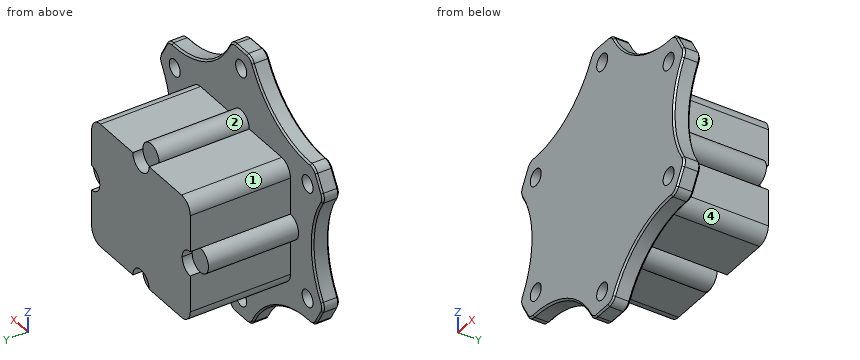
```python
from build123d import *

# Parameters (mm, degrees)
BOSS_EXTRUDE1_DEPTH    = 5
F_10_CLEARANCE_HOLE1_D = 5
FILLET1_R              = 3
CHAMFER1_SIZE          = 0.5
BOSS_EXTRUDE4_DEPTH    = 30
SKETCH5_R              = 3.7
BOSS_EXTRUDE5_DEPTH    = 27


with BuildPart() as part:
    # Sketch1 → Boss-Extrude1 (new body)
    with BuildSketch(Plane.XZ.offset(-227)):
        with BuildLine():
            Line((610.472328875, 48.998023491), (619.472328875, 48.998023491))
            ThreePointArc((619.472328875, 48.998023491), (631.222328875, 61.852197868), (648.22937043, 65.600909174))
            Line((648.22937043, 65.600909174), (652.72937043, 73.395137808))
            ThreePointArc((652.72937043, 73.395137808), (647.472328875, 89.998023491), (652.72937043, 106.600909174))
            Line((652.72937043, 106.600909174), (648.22937043, 114.395137808))
            ThreePointArc((648.22937043, 114.395137808), (631.222328875, 118.143849114), (619.472328875, 130.998023491))
            Line((619.472328875, 130.998023491), (610.472328875, 130.998023491))
            ThreePointArc((610.472328875, 130.998023491), (598.722328875, 118.143849114), (581.71528732, 114.395137808))
            Line((581.71528732, 114.395137808), (577.21528732, 106.600909174))
            ThreePointArc((577.21528732, 106.600909174), (582.472328875, 89.998023491), (577.21528732, 73.395137808))
            Line((577.21528732, 73.395137808), (581.71528732, 65.600909174))
            ThreePointArc((581.71528732, 65.600909174), (598.722328875, 61.852197868), (610.472328875, 48.998023491))
        make_face()
    extrude(amount=-BOSS_EXTRUDE1_DEPTH)

    # #10 Clearance Hole1 (through all)
    with Locations(Plane(origin=(0, 232, 0), x_dir=(1, 0, 0), z_dir=(0, 1, 0))):
        with Locations((614.972328875, -124.998023491), (584.661439743, -72.498023491), (584.661439743, -107.498023491), (614.972328875, -54.998023491), (645.283218008, -107.498023491), (645.283218008, -72.498023491)):
            Hole(F_10_CLEARANCE_HOLE1_D / 2)

    # Fillet1
    fillet1_edges = [part.edges().sort_by_distance(p)[0] for p in [
        (581.71528732, 229.5, 65.600909174),
        (577.21528732, 229.5, 73.395137808),
        (577.21528732, 229.5, 106.600909174),
        (581.71528732, 229.5, 114.395137808),
        (610.472328875, 229.5, 130.998023491),
        (619.472328875, 229.5, 130.998023491),
        (648.22937043, 229.5, 114.395137808),
        (652.72937043, 229.5, 106.600909174),
        (652.72937043, 229.5, 73.395137808),
        (648.22937043, 229.5, 65.600909174),
        (619.472328875, 229.5, 48.998023491),
        (610.472328875, 229.5, 48.998023491),
    ]]
    fillet(fillet1_edges, radius=FILLET1_R)

    # Chamfer1
    chamfer1_edges = [part.edges().sort_by_distance(p)[0] for p in [
        (647.472328875, 227, 89.998023491),
        (647.472328875, 232, 89.998023491),
        (598.722328875, 227, 61.852197868),
        (614.972328875, 227, 48.998023491),
        (631.222328875, 227, 61.852197868),
        (650.47937043, 227, 69.498023491),
        (650.47937043, 227, 110.498023491),
        (631.222328875, 227, 118.143849114),
        (614.972328875, 227, 130.998023491),
        (598.722328875, 227, 118.143849114),
        (579.46528732, 227, 110.498023491),
        (582.472328875, 227, 89.998023491),
        (579.46528732, 227, 69.498023491),
        (581.92524679, 227, 113.911492617),
        (610.786198162, 227, 130.57437066),
        (610.786198162, 227, 49.421676322),
        (577.739116077, 227, 73.335145448),
        (619.158459588, 227, 49.421676322),
        (648.01941096, 227, 113.911492617),
        (619.158459588, 227, 130.57437066),
        (652.205541673, 227, 73.335145448),
        (648.01941096, 227, 66.084554366),
        (581.92524679, 227, 66.084554366),
        (577.739116077, 227, 106.660901535),
        (652.205541673, 227, 106.660901535),
        (650.47937043, 232, 110.498023491),
        (598.722328875, 232, 61.852197868),
        (579.46528732, 232, 69.498023491),
        (582.472328875, 232, 89.998023491),
        (579.46528732, 232, 110.498023491),
        (598.722328875, 232, 118.143849114),
        (614.972328875, 232, 130.998023491),
        (631.222328875, 232, 118.143849114),
        (650.47937043, 232, 69.498023491),
        (631.222328875, 232, 61.852197868),
        (614.972328875, 232, 48.998023491),
        (581.92524679, 232, 113.911492617),
        (610.786198162, 232, 130.57437066),
        (610.786198162, 232, 49.421676322),
        (577.739116077, 232, 73.335145448),
        (619.158459588, 232, 49.421676322),
        (648.01941096, 232, 113.911492617),
        (619.158459588, 232, 130.57437066),
        (652.205541673, 232, 73.335145448),
        (648.01941096, 232, 66.084554366),
        (581.92524679, 232, 66.084554366),
        (577.739116077, 232, 106.660901535),
        (652.205541673, 232, 106.660901535),
    ]]
    chamfer(chamfer1_edges, length=CHAMFER1_SIZE)

    # Sketch4 → Boss-Extrude4 (add)
    with BuildSketch(Plane(origin=(0, 232, 0), x_dir=(1, 0, 0), z_dir=(0, 1, 0))):
        with BuildLine():
            ThreePointArc((611.272328875, -108.698023491), (614.972328875, -104.998023491), (618.672328875, -108.698023491))
            Line((618.672328875, -108.698023491), (633.472328875, -108.698023491))
            ThreePointArc((633.472328875, -108.698023491), (636.300756, -107.526450616), (637.472328875, -104.698023491))
            Line((637.472328875, -104.698023491), (637.472328875, -93.698023491))
            ThreePointArc((637.472328875, -93.698023491), (633.772328875, -89.998023491), (637.472328875, -86.298023491))
            Line((637.472328875, -86.298023491), (637.472328875, -75.298023491))
            ThreePointArc((637.472328875, -75.298023491), (636.300756, -72.469596366), (633.472328875, -71.298023491))
            Line((633.472328875, -71.298023491), (618.672328875, -71.298023491))
            ThreePointArc((618.672328875, -71.298023491), (614.972328875, -74.998023491), (611.272328875, -71.298023491))
            Line((611.272328875, -71.298023491), (596.472328875, -71.298023491))
            ThreePointArc((596.472328875, -71.298023491), (593.64390175, -72.469596366), (592.472328875, -75.298023491))
            Line((592.472328875, -75.298023491), (592.472328875, -86.298023491))
            ThreePointArc((592.472328875, -86.298023491), (595.088623966, -87.381728401), (596.172328875, -89.998023491))
            ThreePointArc((596.172328875, -89.998023491), (595.088623966, -92.614318581), (592.472328875, -93.698023491))
            Line((592.472328875, -93.698023491), (592.472328875, -104.698023491))
            ThreePointArc((592.472328875, -104.698023491), (593.64390175, -107.526450616), (596.472328875, -108.698023491))
            Line((596.472328875, -108.698023491), (611.272328875, -108.698023491))
        make_face()
    extrude(amount=BOSS_EXTRUDE4_DEPTH)

    # Sketch5 → Boss-Extrude5 (add)
    with BuildSketch(Plane(origin=(0, 232, 0), x_dir=(1, 0, 0), z_dir=(0, 1, 0))):
        with Locations((614.972328875, -71.298023491)):
            Circle(SKETCH5_R)
        with Locations((637.472328875, -89.998023491)):
            Circle(SKETCH5_R)
        with Locations((614.972328875, -108.698023491)):
            Circle(SKETCH5_R)
        with Locations((592.472328875, -89.998023491)):
            Circle(SKETCH5_R)
    extrude(amount=BOSS_EXTRUDE5_DEPTH)


solid = part.part
```
Geometry: final body of the model. Coordinates: model frame, mm. Face numbers are marked on the shaded views. A direction names the side the tool comes from. Round coordinates to 2 decimals unless told otherwise and drop trailing zeros. Write each loop counter-clockwise with the first axis right and the second up, starting at its lowest first coordinate (ties: lowest second). Pieces come first, ordered by that corner, then holes.
Item 1: Section query B-B (x = 613.5). Return loops of the section in (y, z), plus the area to 3 significant figures.
Item 2: Section query A-A (y = 234.5). Return loops of the section in (x, z).
Item 3: Material intervals for L1, parallel to Y at x = 644.5, z = 85; L2, parallel to X at y = 233, z = 99.5; L3, parallel to Z at x = 628, y = 244, sorted ascending.
Item 4: Set-up query: the marked faces 1, 2, 3 and 4. Return all of +Z, -Z, +X, -X, +Y, -Y with unobstructed straight access to the full face (end or side cutting, diameter ignored); none if empty.
Item 5: Pin query (flat end, axial travel): P1, Ø8, axis at x = 584.66, z = 72.5, coming from the -Y side; P2, Ø5, axis at y = 231, z = 77.5, coming from the -X side; P3, Ø16.5, axis at x = 629, y = 241, coming from the -Z side; P4, Ø3.5, axis at x = 613.5, z = 108, coming from the +Y side. Return the tip coordinate at first contact, or that it passes through.
Completed:
1. outline: (227, 49.5) - (227.5, 49) - (231.5, 49) - (232, 49.5) - (232, 52.98) - (227, 52.98) - close; (227, 57.02) - (232, 57.02) - (232, 67.9) - (259, 67.9) - (259, 74.69) - (262, 74.69) - (262, 105.3) - (259, 105.3) - (259, 112.09) - (232, 112.09) - (232, 122.98) - (227, 122.98) - close; (227, 127.02) - (232, 127.02) - (232, 130.5) - (231.5, 131) - (227.5, 131) - (227, 130.5) - close
1. area: 1,650 mm2
2. outline: (592.47, 75.3) arc R4 ccw to (596.47, 71.3) - (611.27, 71.3) arc R3.7 ccw to (618.67, 71.3) - (633.47, 71.3) arc R4 ccw to (637.47, 75.3) - (637.47, 86.3) arc R3.7 ccw to (637.47, 93.7) - (637.47, 104.7) arc R4 ccw to (633.47, 108.7) - (618.67, 108.7) arc R3.7 ccw to (611.27, 108.7) - (596.47, 108.7) arc R4 ccw to (592.47, 104.7) - (592.47, 93.7) arc R3.7 ccw to (592.47, 86.3) - close
3. L1: y = 227 to 232
3. L2: x = 592.47 to 637.47
3. L3: z = 71.3 to 108.7
4. face 1: +Z, -X, +Y
4. face 2: +Z, +Y
4. face 3: +Z, +X, +Y
4. face 4: -Z, +X, +Y
5. P1: stops at y = 227
5. P2: stops at x = 578.27
5. P3: stops at z = 71.3
5. P4: stops at y = 259
